from build123d import *

# Parameters (mm, degrees)
SKETCH1_R           = 57.5
BOSS_EXTRUDE1_DEPTH = 5
BOSS_EXTRUDE2_DEPTH = 40.75
CUT_EXTRUDE1_DEPTH  = 22.25
CUT_EXTRUDE2_DEPTH  = 4.5
CUT_EXTRUDE3_DEPTH  = 12
SKETCH7_R           = 9
CUT_EXTRUDE5_DEPTH  = 2
SKETCH8_R           = 1.3
CUT_EXTRUDE6_DEPTH  = 7.5
SKETCH10_R          = 3.75
CUT_EXTRUDE7_DEPTH  = 14
SKETCH11_R          = 3.75
CUT_EXTRUDE8_DEPTH  = 2
CUT_EXTRUDE9_REACH  = 66.458
SKETCH12_R          = 0.85
BOSS_EXTRUDE3_DEPTH = 3
FILLET1_R           = 0.5


with BuildPart() as part:
    # Sketch1 → Boss-Extrude1 (new body)
    with BuildSketch(Plane(origin=(0, 0, 0), x_dir=(1, 0, 0), z_dir=(0, 1, 0))):
        Circle(SKETCH1_R)
    extrude(amount=BOSS_EXTRUDE1_DEPTH)

    # Sketch2 → Boss-Extrude2 (add, symmetric)
    with BuildSketch(Plane.XY):
        with BuildLine():
            Line((-35, 5), (-35, 13))
            ThreePointArc((-35, 13), (-32.785945694, 23.285945694), (-26.535945694, 31.75))
            Line((-26.535945694, 31.75), (3.464054306, 58.207513111))
            ThreePointArc((3.464054306, 58.207513111), (37.67766953, 57.13518264), (38.75, 22.921567416))
            ThreePointArc((38.75, 22.921567416), (35.9687848, 18.303300859), (35, 13))
            Line((35, 13), (35, 5))
            Line((35, 5), (-35, 5))
        make_face()
    extrude(amount=BOSS_EXTRUDE2_DEPTH, both=True)

    # Sketch4 → Cut-Extrude1 (cut, symmetric)
    with BuildSketch(Plane.XY):
        with BuildLine():
            Line((3.464054306, 58.207513111), (-26.535945694, 31.75))
            ThreePointArc((-26.535945694, 31.75), (-32.785945694, 23.285945694), (-35, 13))
            Line((-35, 13), (-35, 5))
            Line((-35, 5), (35, 5))
            Line((35, 5), (35, 13))
            ThreePointArc((35, 13), (35.9687848, 18.303300859), (38.75, 22.921567416))
            ThreePointArc((38.75, 22.921567416), (37.67766953, 57.13518264), (3.464054306, 58.207513111))
        make_face()
    extrude(amount=CUT_EXTRUDE1_DEPTH, both=True, mode=Mode.SUBTRACT)

    # Sketch5 → Cut-Extrude2 (cut)
    with BuildSketch(Plane.XY.offset(40.75)):
        with BuildLine():
            Line((5.448367789, 55.957513111), (-19.449111825, 34))
            ThreePointArc((-19.449111825, 34), (-26.449111825, 24.520259177), (-28.928852648, 13))
            Line((-28.928852648, 13), (-28.928852648, 5))
            Line((-28.928852648, 5), (29.071147352, 5))
            Line((29.071147352, 5), (29.071147352, 13))
            ThreePointArc((29.071147352, 13), (30.242434209, 18.064703602), (33.518438806, 22.100905947))
            ThreePointArc((33.518438806, 22.100905947), (36.936184172, 53.499082314), (5.448367789, 55.957513111))
        make_face()
    cut_extrude2 = extrude(amount=-CUT_EXTRUDE2_DEPTH, mode=Mode.SUBTRACT)

    # Mirror1: Cut-Extrude2 across plane
    add(cut_extrude2.mirror(Plane.XY), mode=Mode.SUBTRACT)

    # Sketch6 → Cut-Extrude3 (cut)
    with BuildSketch(Plane.XY.offset(36.25)):
        Polygon((20.554902808, 53.946891388), (-10.195097192, 26.82794045), (3.695097192, 11.07794045), (34.445097192, 38.196891388), align=None)
    extrude(amount=-CUT_EXTRUDE3_DEPTH, mode=Mode.SUBTRACT)

    # Sketch7 → Cut-Extrude5 (cut)
    with BuildSketch(Plane.XY.offset(24.25)):
        with Locations((19.625, 39.126794197)):
            Circle(SKETCH7_R)
    extrude(amount=-CUT_EXTRUDE5_DEPTH, mode=Mode.SUBTRACT)

    # Sketch8 → Cut-Extrude6 (cut)
    with BuildSketch(Plane.XY.offset(36.25)):
        with Locations((27.042810861, 52.335355134)):
            Circle(SKETCH8_R)
        with Locations((33.657189139, 44.835355134)):
            Circle(SKETCH8_R)
        with Locations((-9.407189139, 20.189476704)):
            Circle(SKETCH8_R)
        with Locations((-2.792810861, 12.689476704)):
            Circle(SKETCH8_R)
    extrude(amount=-CUT_EXTRUDE6_DEPTH, mode=Mode.SUBTRACT)

    # Sketch10 → Cut-Extrude7 (cut)
    with BuildSketch(Plane.XY.offset(-22.25)):
        with Locations((19.625, 39.126794197)):
            Circle(SKETCH10_R)
    extrude(amount=-CUT_EXTRUDE7_DEPTH, mode=Mode.SUBTRACT)

    # Sketch11 → Cut-Extrude8 (cut)
    with BuildSketch(Plane.XZ):
        Circle(SKETCH11_R)
    extrude(amount=-CUT_EXTRUDE8_DEPTH, mode=Mode.SUBTRACT)

    # Sketch12 → Cut-Extrude9 (cut, up to next)
    with BuildSketch(Plane.XZ, mode=Mode.PRIVATE) as cut_extrude9_sk1:
        with Locations((7, 0)):
            Circle(SKETCH12_R)
    cut_extrude9_tool1 = extrude(cut_extrude9_sk1.sketch, amount=-CUT_EXTRUDE9_REACH, mode=Mode.PRIVATE) & part.part
    add(cut_extrude9_tool1.solids().sort_by_distance((7, 0, 0))[0], mode=Mode.SUBTRACT)
    # Sketch12 → Cut-Extrude9 (cut, up to next)
    with BuildSketch(Plane.XZ, mode=Mode.PRIVATE) as cut_extrude9_sk2:
        with Locations((-7, 0)):
            Circle(SKETCH12_R)
    cut_extrude9_tool2 = extrude(cut_extrude9_sk2.sketch, amount=-CUT_EXTRUDE9_REACH, mode=Mode.PRIVATE) & part.part
    add(cut_extrude9_tool2.solids().sort_by_distance((-7, 0, 0))[0], mode=Mode.SUBTRACT)

    # Sketch13 → Boss-Extrude3 (add, symmetric)
    with BuildSketch(Plane(origin=(0, 0, 0), x_dir=(0, 0, -1), z_dir=(1, 0, 0))):
        with BuildLine():
            Line((22.25, 5), (22.25, 10))
            ThreePointArc((22.25, 10), (21.371320344, 12.121320344), (19.25, 13))
            Line((19.25, 13), (9.25, 13))
            ThreePointArc((9.25, 13), (7.128679656, 12.121320344), (6.25, 10))
            Line((6.25, 10), (6.25, 5))
            Line((6.25, 5), (10.25, 5))
            Line((10.25, 5), (10.25, 9))
            Line((10.25, 9), (18.25, 9))
            Line((18.25, 9), (18.25, 5))
            Line((18.25, 5), (22.25, 5))
        make_face()
    extrude(amount=BOSS_EXTRUDE3_DEPTH, both=True)

    # Fillet1
    fillet1_edges = [part.edges().sort_by_distance(p)[0] for p in [
        (-3, 5, -20.25),
        (0, 5, -18.25),
        (-3, 5, -8.25),
        (0, 5, -6.25),
        (0, 5, -10.25),
        (3, 5, -20.25),
        (3, 5, -8.25),
    ]]
    fillet(fillet1_edges, radius=FILLET1_R)


solid = part.part
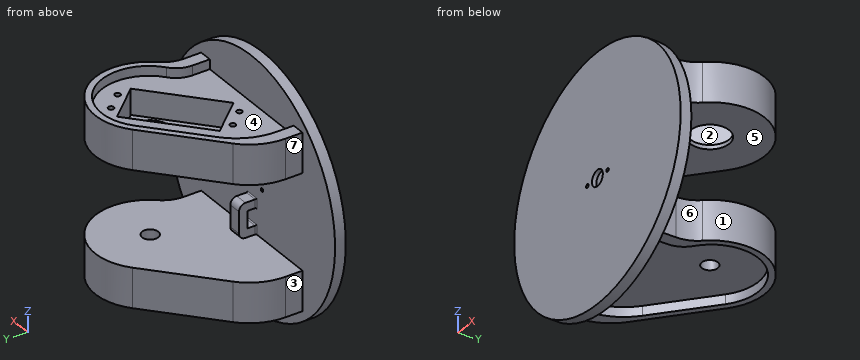
Source: CAD feature listing. Evaluate the final solid. Frame: model axes, mm. Face numbers are marked on the shaded views. A direction names the side the tool comes from. Give positions to 0.01 mm unless a question says otherwise; leave off trailing zeros. Write each loop counter-clockwise with the first axis right and the second up, starting at its lowest first coordinate (ties: lowest second). Pieces come first, ordered by that corner, then holes. Notation, with made-up numbers: M 5,63 L 64,63 A29 ccw 64,95 Z; hole C 17.5,57 d8. An arc over 180 degrees is marked long. Return JSON: item names as keys, results as strings. Group by question number.
1) First-contact query: pin 1 Ø1.3 at (x, y) = (26.5, 51.5) entering from +Z; pin 2 Ø2 at (x, z) = (-20.5, -11.5) entering from +Y; pin 3 Ø5 at (x, z) = (0, -15) entering from +Y. Flat tips, straight axial feed; report the tip coordinate or a pass-through.
2) Cut plane B-B, the plane z = 14. Output: boundary loops of the cut face in (x, y), then the cut area to 3 significant figures.
3) Cut plane A-A, the plane x = -43.5. Output: boundary loops of the cut face in (y, z).
4) Set-up query: the marked faces 4, 5, 6 and 7. Return all of +Z, -Z, +X, -X, +Y, -Y with unobstructed straight access to the full face (end or side cutting, diameter ignored); none if empty.
5) Draft query along X for the marked faces 1, 2 and 3. Return one class per face: released by +X, released by -X, zero draft, split by the parting line, or undercut.
6) Ray query, L1, parallel to Z at x = 38.5, y = 31.5; L2, parallel to Z at x = 34, y = 58.5; L3, parallel to Y at x = -15, z = 17. Return the intervals inside material, ascending.
Data:
{
 "1": {"pin 1": "stops at z = 36.25", "pin 2": "stops at y = 5", "pin 3": "stops at y = 13"},
 "2": {"outline": "M -55.77,0 L 55.77,0 L 55.77,5 L -55.77,5 Z", "area": "558 mm²"},
 "3": {"outline": "M 0,-37.6 L 5,-37.6 L 5,37.6 L 0,37.6 Z"},
 "4": {"face 4": "+Z", "face 5": "+X, -X, +Y", "face 6": "+Z, -Z, +X", "face 7": "+Z, -Z, -X, +Y"},
 "5": {"face 1": "split by the parting line", "face 2": "undercut", "face 3": "released by -X"},
 "6": {"L1": "z = -36.25 to -22.25, 22.25 to 36.25", "L2": "z = -40.75 to -22.25, 22.25 to 40.75", "L3": "y = 0 to 5"}
}
